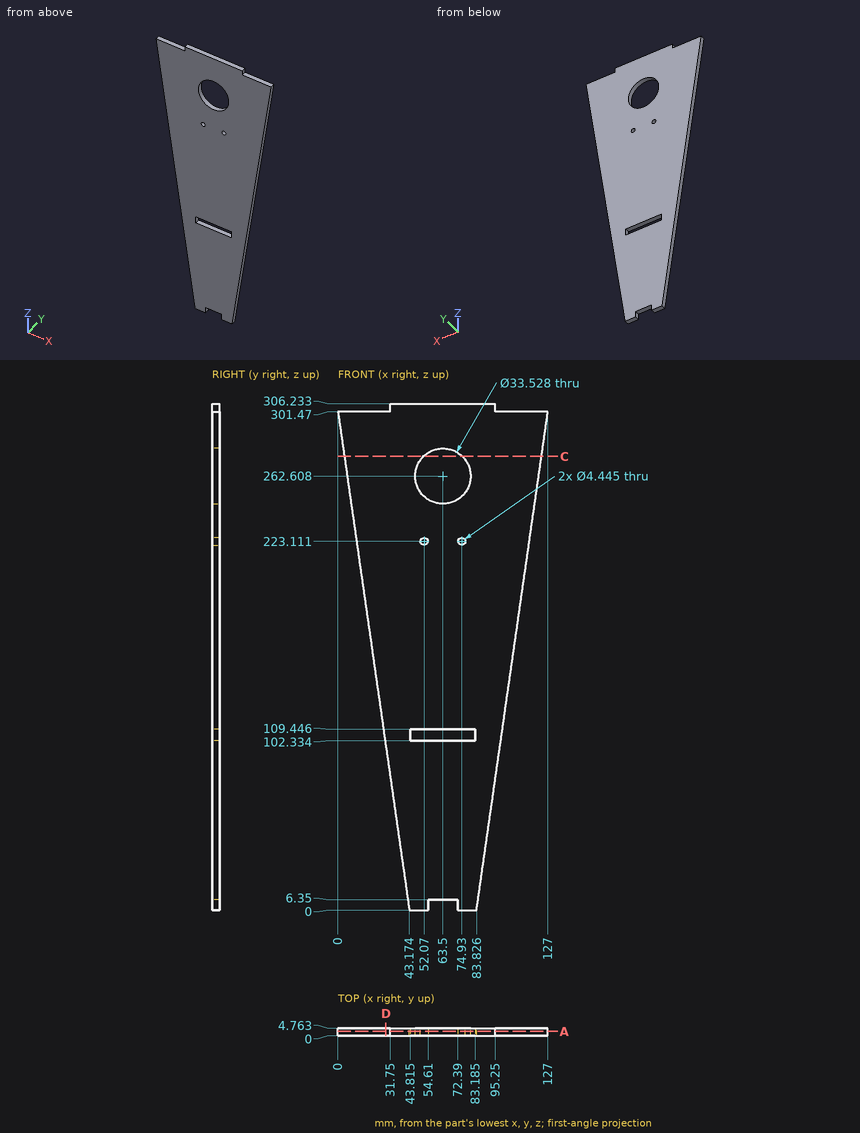
Check sheet for the drawn part. Datum: minimum x, y, z corner. Units: mm. Give positions to 0.01 mm unless a question says otherwise; leave off trailing zeros. Write each loop counter-clockwise with the first axis right and the second up, starting at its lowest first coordinate (ties: lowest second). Pieces come first, ordered by that corner, then holes. Notation, with made-up numbers: (-38, 41.25) -> (-27, 41.25) arc R28 cw to (-27, 62.25) -> close; hole circle Ø6 at (24.5, 64). An arc over 180 degrees is marked (long way). Use one line per item in the form item = value. Start each with the question number.
1. Section check D-D (x = 29). Record the cut outline in (y, z).
2. Thickness scan on line 1 along Z through (x, y) = (74.93, 1.25) (1 decimal); line 2 along X through (y, z) = (1.5, 222) (1 decimal); line 3 along X through (y, z) = (2.1, 213). Record the ranges inside material, lowest first. Write a range as from..to.
3. Go/stop test with flat-tipped pins: P1, Ø2.5, axis at x = 12, y = 1.5, coming from the +Z side; P2, Ø2, axis at x = 67, y = 3.5, coming from the -Z side. Record where each tip stops, or that it passes through.
4. Section check C-C (z = 274.5). Record the cut outline in (x, y) (1 decimal).
5. Section check A-A (y = 2.8). Count the separate pieces of the cut face and the enclosed holes in it, and give its area (3 significant figures).
Conclusion:
q1.outline = (0, 98.97) -> (4.76, 98.97) -> (4.76, 301.47) -> (0, 301.47) -> close
q2.line_1 = 0..102.3, 109.4..220.9, 225.3..250.3, 274.9..306.2
q2.line_2 = 11.4..50.1, 54..73, 76.9..115.6
q2.line_3 = 12.67..114.33
q3.P1 = 301.47
q3.P2 = 6.35
q4.outline = (3.9, 0) -> (51.7, 0) -> (51.7, 4.8) -> (3.9, 4.8) -> close; (75.3, 0) -> (123.1, 0) -> (123.1, 4.8) -> (75.3, 4.8) -> close
q5.separate_pieces = 1
q5.enclosed_holes = 4
q5.area = 24,300 mm²
